Here's how the part is built. I have some questions about the finished solid (model axes, mm). A direction names the side the tool comes from. Give positions to 0.01 mm unless a question says otherwise; leave off trailing zeros. Write each loop counter-clockwise with the first axis right and the second up, starting at its lowest first coordinate (ties: lowest second). Pieces come first, ordered by that corner, then holes. Notation, with made-up numbers: (-30.75, 10) - (-14.75, 10) arc R22 ccw to (-14.75, 37) - close; hole circle Ø4 at (43.25, 75.5). An arc over 180 degrees is marked (long way). Use a Markdown table: item, result.
```python
from build123d import *

# Parameters (mm, degrees)
F0_W      = 109.22
F0_H      = 25.4
F1_DEPTH  = 90.17
F2_W      = 105.22204
F2_H      = 86.17204
F3_DEPTH  = 23.368
F6_D      = 3.556
F10_R     = 2.7904831324
F11_DEPTH = 25.4
F13_D     = 3.175
F13_DEPTH = 12.7
F13_TIP   = 0.9538662327
F14_W     = 2.5
F14_H     = 7.5
F15_DEPTH = 5.08
F17_D     = 3.175
F17_DEPTH = 12.7
F17_TIP   = 0.9538662327
F19_D     = 3.175
F19_DEPTH = 12.7
F19_TIP   = 0.9538662327
F21_D     = 3.175
F21_DEPTH = 12.7
F21_TIP   = 0.9538662327


# Not quite as in the source:
# - a feature of the source that left no trace in its solid (it failed there, or was rolled back) is left out
# - a feature names something its author has since deleted; it is built from what else it names


with BuildPart() as f1:
    # F0 (on Front) → F1 (new body)
    with BuildSketch(Plane.XZ):
        Rectangle(F0_W, F0_H)
    extrude(amount=F1_DEPTH)

    # F2 (on face) → F3 (cut)
    with BuildSketch(Plane.XY.offset(12.7)):
        with Locations((0, -45.085)):
            Rectangle(F2_W, F2_H)
    extrude(amount=-F3_DEPTH, mode=Mode.SUBTRACT)

    # F6 (through all)
    with Locations(Plane.XY.offset(-10.668)):
        with Locations((-34.2227290702, -12.5292580739), (31.5179094365, -9.3542580739), (31.5179094365, -57.6142580739)):
            Hole(F6_D / 2)

    # F10 (on face) → F11 (cut)
    with BuildSketch(Plane(origin=(0, 0, -12.7), x_dir=(1, 0, 0), z_dir=(0, 0, -1))):
        with Locations((-37.1684581041, 13.9195527881)):
            Circle(F10_R)
    extrude(amount=F11_DEPTH, mode=Mode.SUBTRACT)

    # F13
    with Locations(Plane.XZ.offset(90.17)):
        with Locations((50.546, 10.668), (50.546, -7.112)):
            Hole(F13_D / 2, depth=F13_DEPTH)
            with Locations((0, 0, -(F13_DEPTH + F13_TIP / 2))):  # 118° drill point
                Cone(0, F13_D / 2, F13_TIP, mode=Mode.SUBTRACT)

    # F14 (on face) → F15 (cut)
    with BuildSketch(Plane.YZ.offset(54.61)):
        with Locations((-78.2630409374, 1.6418104)):
            Rectangle(F14_W, F14_H)
    extrude(amount=-F15_DEPTH, mode=Mode.SUBTRACT)

    # F17
    with Locations(Plane(origin=(0, 0, 0), x_dir=(1, 0, 0), z_dir=(0, 1, 0))):
        with Locations((-6.2431572373, -8.382), (-45.6131572373, -8.382)):
            Hole(F17_D / 2, depth=F17_DEPTH)
            with Locations((0, 0, -(F17_DEPTH + F17_TIP / 2))):  # 118° drill point
                Cone(0, F17_D / 2, F17_TIP, mode=Mode.SUBTRACT)

    # F19
    with Locations(Plane(origin=(-54.61, 0, 0), x_dir=(0, -1, 0), z_dir=(-1, 0, 0))):
        with Locations((30.48, 8.382)):
            Hole(F19_D / 2, depth=F19_DEPTH)
            with Locations((0, 0, -(F19_DEPTH + F19_TIP / 2))):  # 118° drill point
                Cone(0, F19_D / 2, F19_TIP, mode=Mode.SUBTRACT)

    # F21
    with Locations(Plane.XZ.offset(90.17)):
        with Locations((-30.2895, 8.001), (-41.91, 3.7953188), (-18.669, 3.7953188)):
            Hole(F21_D / 2, depth=F21_DEPTH)
            with Locations((0, 0, -(F21_DEPTH + F21_TIP / 2))):  # 118° drill point
                Cone(0, F21_D / 2, F21_TIP, mode=Mode.SUBTRACT)


solid = f1.part
```
Item 1: If we section it at B-B, the plane x = -41.91: Write out the boundary of the cut face in (y, z), plus the area to 3 significant figures.
Values:
| item | result |
|---|---|
| outline | (-90.17, -12.7) - (0, -12.7) - (0, 12.7) - (-2, 12.7) - (-2, -10.67) - (-88.17, -10.67) - (-88.17, 2.21) - (-90.17, 2.21) - close; (-90.17, 5.38) - (-88.17, 5.38) - (-88.17, 12.7) - (-90.17, 12.7) - close |
| area | 270 mm2 |
Item 2: Thinking about a two-plate mould opening in Z: for faces 1 (the flat face through (-1, -44, -10.668)), 2 (the cylindrical face through (-31.02, -89.16, 6.59)), 3 (the flat face through (-1, -90.17, 0)), which applies, +Z half, -Z half, draft (parallel to the pull), parting line (faces both ways), or undercut?
Values:
| item | result |
|---|---|
| face 1 | +Z half |
| face 2 | undercut |
| face 3 | draft |
Item 3: I need wall thicknesses on line 1 along X through (y, z) = (-5.5, -7); line 2 along Y through (x, z) = (-5.5, 5.75); line 3 along Z through (x, y) = (-33, -67.5). Which ranges of each line are inside material? Lowest first, please. Write a range as [from, to].
Values:
| item | result |
|---|---|
| line 1 | x = [-54.61, -52.61], [52.61, 54.61] |
| line 2 | y = [-90.17, -88.17], [-2, 0] |
| line 3 | z = [-12.7, -10.67] |
Item 4: Will these pins go through, and if not, where does the flat tip stop? pin 1 Ø5 at (x, y) = (-17.5, -17.5) entering from +Z; pin 2 Ø4.5 at (x, y) = (31.52, -9.35) entering from -Z; pin 3 Ø1.9 at (x, z) = (-18.67, 3.8) entering from -Y.
Values:
| item | result |
|---|---|
| pin 1 | stops at z = -10.67 |
| pin 2 | stops at z = -12.7 |
| pin 3 | stops at y = -2 |
Item 5: If we section it at C-C, the plane z = -4.25: Write out the boundary of the cut face in (x, y), plus the area to 3 significant figures.
Values:
| item | result |
|---|---|
| outline | (-54.61, -90.17) - (54.61, -90.17) - (54.61, 0) - (-54.61, 0) - close; hole (-52.61, -88.17) - (52.61, -88.17) - (52.61, -2) - (-52.61, -2) - close |
| area | 781 mm2 |
Item 6: If we section it at D-D, the plane y = -67: Write out the boundary of the cut face in (x, z), plus the area to 3 significant figures.
Values:
| item | result |
|---|---|
| outline | (-54.61, -12.7) - (54.61, -12.7) - (54.61, 12.7) - (52.61, 12.7) - (52.61, -10.67) - (-52.61, -10.67) - (-52.61, 12.7) - (-54.61, 12.7) - close |
| area | 315 mm2 |
Item 7: If we section it at A-A, the plane y = -30.48: Write out the boundary of the cut face in (x, z), plus the area to 3 significant figures.
Values:
| item | result |
|---|---|
| outline | (-54.61, -12.7) - (54.61, -12.7) - (54.61, 12.7) - (52.61, 12.7) - (52.61, -10.67) - (-52.61, -10.67) - (-52.61, 6.79) - (-54.61, 6.79) - close; (-54.61, 9.97) - (-52.61, 9.97) - (-52.61, 12.7) - (-54.61, 12.7) - close |
| area | 309 mm2 |
Item 8: For faces 4 (the flat face through (-52.611, -46, 1)), 5 (the cylindrical face through (-53.597, -28.966, 8.859)), 6 (the cylindrical face through (-6.036, -1.013, 6.808)), 7 (the cylindrical face through (52.13, -89.16, 10.74)), which set-ups out of +Z, -Z, +X, -X, +Y, -Y let a thin tool reach every point of the face, with its end or its side?
Values:
| item | result |
|---|---|
| face 4 | +Z |
| face 5 | -X |
| face 6 | +Y |
| face 7 | -Y |
